Autodesk Inventor part; units mm, degrees
ref_plane "РабПлоскость1" through (0, 0, 30) normal (0, 0, 1) x (1, 0, 0)
ref_plane "YZ Plane" through (0, 0, 0) normal (1, 0, 0) x (0, 1, 0)
ref_plane "XZ Plane" through (0, 0, 0) normal (0, 1, 0) x (-1, 0, 0)
sketch "Эскиз1" plane through (0, 0, 0) normal (0, 0, 1) x (1, 0, 0)
  line L0 (0, 0) -> (0, 20)
  line L1 (0, 20) -> (2.8284, 22.8284)
  line L2 (0, 0) -> (15, 0)
  line L3 (15, 0) -> (15, 20)
  line L4 (15, 20) -> (12.1716, 22.8284)
  line L5 (12.1716, 22.8284) -> (2.8284, 22.8284)
  dimension "d0" = 20
  dimension "d1" = 4
  dimension "d2" = 135
  dimension "d3" = 15
  dimension "d4" = 4
  dimension "d5" = 135
revolve "Вращение1" add sketch "Эскиз1" angle 360 about axis through (0, 0, 0) along (1, 0, 0)
sketch "Эскиз2" plane through (0, 0, 0) normal (-1, 0, 0) x (0, 0, 1)
  point P0 (0, 0)
  point P1 (0, 18)
  point P2 (-15.5885, 9)
  point P3 (-15.5885, -9)
  point P4 (0, -18)
  point P5 (15.5885, -9)
  point P6 (15.5885, 9)
  dimension "d7" = 18
  dimension "d10" = 360
hole "Отверстие1" at (0, 18, 0) at (0, 9, -15.5885) at (0, -9, -15.5885) at (0, -18, 0) at (0, -9, 15.5885) at (0, 9, 15.5885) direction (1, 0, 0) diameter 4 depth 4
sketch "Эскиз3" plane through (0, 0, 0) normal (0, 0, 1) x (1, 0, 0)
  line L0 (0, 0) -> (0, 8)
  line L1 (0, 8) -> (0.7, 7.3)
  line L2 (0, 8) -> (0.9899, 8) construction
  line L3 (0.7, 7.3) -> (6.643, 7.3)
  line L4 (6.643, 7.3) -> (6.643, 8)
  line L5 (6.643, 8) -> (7.343, 8)
  line L6 (7.343, 8) -> (7.343, 7.3)
  line L7 (7.343, 7.3) -> (10, 0)
  line L8 (10, 0) -> (0, 0)
  point P0 (0, 0)
  dimension "d19" = 45
  dimension "d20" = 70
  dimension "d21" = 8
  dimension "d22" = 0.7
  dimension "d23" = 0.7
  dimension "d24" = 10
revolve "Вращение2" cut sketch "Эскиз3" angle 360 about axis through (10, 0, 0) along (-1, 0, 0)
ref_plane "РабПлоскость1" through (0, 0, 30) normal (0, 0, 1) x (1, 0, 0)
sketch "Эскиз4" plane through (0, 0, 30) normal (0, 0, 1) x (1, 0, 0)
  line L0 (15, -20) -> (15, 20) construction
  line L1 (15, 1.5) -> (10.5, 1.5)
  line L2 (10.5, 1.5) -> (10.5, -1.5)
  line L3 (10.5, -1.5) -> (15, -1.5)
  line L4 (15, -1.5) -> (15, 1.5)
  point P0 (0, 0)
  point P1 (15, 0)
  point P2 (15, 0)
  dimension "d27" = 4.5
  dimension "d28" = 3
extrude "Выдавливание1" cut sketch "Эскиз4" against normal through all
properties part number "711137"
The model under review builds one solid part; all positions refer to its coordinate system, in mm. A direction names the side the tool comes from. Give positions to 0.01 mm unless a question says otherwise; leave off trailing zeros. Loops run counter-clockwise (first coordinate to the right, second up) from the corner with the lowest first, then second, coordinate; pieces in that order, holes last. Notation, with made-up numbers: (-37, -37.75) -> (-5, -37.75) arc R21 ccw to (-5, -19.75) -> close; hole circle Ø3 at (24.25, 85). An arc over 180 degrees is marked (long way). Use CSV: the item, a comma, the result in double quotes.
1. For P1, Ø3, axis at x = 4.5, z = 11.5, coming from the +Y side; P2, Ø1.5, axis at y = 0, z = -6.5, coming from the +X side; P3, Ø3.5, axis at y = -9, z = -15.59, coming from the -X side, all flat-tipped, find the tip position at first contact; note any pin that passes through.
Result:
P1,"stops at y = 20.52"
P2,"stops at x = 10.5"
P3,"stops at x = 4"
2. The part is to be moulded in two halves that separate along Z. For faces 4 (the face through (7.435, -4.949, 22.286)), 5 (the face through (4, -18, 0)), 6 (the face through (15, 9, 0)), say which applies: +Z half, -Z half, draft (parallel to the pull), parting line (faces both ways), or undercut.
Result:
face 4,"parting line"
face 5,"undercut"
face 6,"draft"
3. Consider section A-A, the plane x = 8. Write out the cut boundary in (y, z).
Result:
outline,"circle Ø45.66 at (0, 0); hole circle Ø10.99 at (0, 0)"
4. To check wall thickness, follow probe 1 along Z at (x, y) = (1.85, 9); probe 2 along Z at (x, y) = (5.2, 0); probe 3 along Y at (x, z) = (7.2, 0). State the ranges of each line that lie inside material, in increasing order. Write a range as from..to.
Result:
probe 1,"z = -19.91..-17.59, -13.59..13.59, 17.59..19.91"
probe 2,"z = -22.83..-7.3, 7.3..22.83"
probe 3,"y = -22.83..-8, 8..22.83"
5. Machinability: for faces 1 (the face through (2.03, 7.31, 16.66)), 2 (the face through (6.643, 2.3, 7.1)), 3 (the face through (10.5, 0, 0)), which of the approach directions +Z, -Z, +X, -X, +Y, -Y give a long, thin tool a straight path to every point of the face, cutting with its end or side? Answer none if there is none.
Result:
face 1,"-X"
face 2,"none"
face 3,"+Z, -Z, +X"
